Design review of the part built by this model. Coordinates are the model's own, in mm. Round coordinates to 2 decimals unless told otherwise and drop trailing zeros. Loops run counter-clockwise (first coordinate to the right, second up) from the corner with the lowest first, then second, coordinate; pieces in that order, holes last. Notation, with made-up numbers: M 37,-2.75 L 79,-2.75 A30 ccw 79,34.25 Z; hole C 58,45 d9. An arc over 180 degrees is marked long. Use a Markdown table: item, result.
from build123d import *

# Parameters (mm, degrees)
BOSS_EXTRUDE1_DEPTH = 3
FILLET1_R           = 5
CUT_EXTRUDE1_DEPTH  = 3
SKETCH3_W           = 3
SKETCH3_H           = 185.5
BOSS_EXTRUDE2_DEPTH = 5
BOSS_EXTRUDE3_DEPTH = 3
BOSS_EXTRUDE4_DEPTH = 3


with BuildPart() as part:
    # Sketch1 → Boss-Extrude1 (new body)
    with BuildSketch(Plane.XY):
        with BuildLine():
            Line((-23.5, 139.962429423), (-23.5, 114.5))
            Line((-23.5, 114.5), (3, 114.5))
            Line((3, 114.5), (3, 54.962429423))
            Line((3, 54.962429423), (-23.5, 54.962429423))
            Line((-23.5, 54.962429423), (-23.5, 29.5))
            Line((-23.5, 29.5), (3, 29.5))
            Line((3, 29.5), (3, -30.037570577))
            Line((3, -30.037570577), (-23.5, -30.037570577))
            Line((-23.5, -30.037570577), (-23.5, -55.5))
            Line((-23.5, -55.5), (3, -55.5))
            Line((3, -55.5), (3, -75.25))
            ThreePointArc((3, -75.25), (-20, -98.25), (-43, -75.25))
            Line((-43, -75.25), (-43, 160.25))
            ThreePointArc((-43, 160.25), (-20, 183.25), (3, 160.25))
            Line((3, 160.25), (3, 139.962429423))
            Line((3, 139.962429423), (-23.5, 139.962429423))
        make_face()
    extrude(amount=BOSS_EXTRUDE1_DEPTH)

    # Fillet1
    fillet1_edges = [part.edges().sort_by_distance(p)[0] for p in [
        (-23.5, 139.962429423, 1.5),
        (-23.5, 114.5, 1.5),
        (-23.5, 54.962429423, 1.5),
        (-23.5, 29.5, 1.5),
        (-23.5, -30.037570577, 1.5),
        (-23.5, -55.5, 1.5),
    ]]
    fillet(fillet1_edges, radius=FILLET1_R)

    # Sketch2 → Cut-Extrude1 (cut)
    with BuildSketch(Plane.XY.offset(3)):
        with BuildLine():
            Line((-31.934718262, 161.5), (-8.065281738, 161.5))
            ThreePointArc((-8.065281738, 161.5), (-8, 160.25), (-8.065281738, 159))
            Line((-8.065281738, 159), (-31.934718262, 159))
            ThreePointArc((-31.934718262, 159), (-32, 160.25), (-31.934718262, 161.5))
        make_face()
        with BuildLine():
            Line((-31.399013115, 164), (-8.600986885, 164))
            ThreePointArc((-8.600986885, 164), (-9.106587826, 165.283246588), (-9.756099376, 166.5))
            Line((-9.756099376, 166.5), (-30.243900624, 166.5))
            ThreePointArc((-30.243900624, 166.5), (-30.893412174, 165.283246588), (-31.399013115, 164))
        make_face()
        with BuildLine():
            Line((-28.212033853, 169), (-11.787966147, 169))
            ThreePointArc((-11.787966147, 169), (-20, 172.25), (-28.212033853, 169))
        make_face()
        with BuildLine():
            Line((-28.212033853, 151.5), (-11.787966147, 151.5))
            ThreePointArc((-11.787966147, 151.5), (-20, 148.25), (-28.212033853, 151.5))
        make_face()
        with BuildLine():
            Line((-30.243900624, 154), (-9.756099376, 154))
            ThreePointArc((-9.756099376, 154), (-9.106587826, 155.216753412), (-8.600986885, 156.5))
            Line((-8.600986885, 156.5), (-31.399013115, 156.5))
            ThreePointArc((-31.399013115, 156.5), (-30.893412174, 155.216753412), (-30.243900624, 154))
        make_face()
        with BuildLine():
            Line((-31.399013115, -71.5), (-8.600986885, -71.5))
            ThreePointArc((-8.600986885, -71.5), (-9.106587826, -70.216753412), (-9.756099376, -69))
            Line((-9.756099376, -69), (-30.243900624, -69))
            ThreePointArc((-30.243900624, -69), (-30.893412174, -70.216753412), (-31.399013115, -71.5))
        make_face()
        with BuildLine():
            Line((-28.212033853, -66.5), (-11.787966147, -66.5))
            ThreePointArc((-11.787966147, -66.5), (-20, -63.25), (-28.212033853, -66.5))
        make_face()
        with BuildLine():
            Line((-31.934718262, -74), (-8.065281738, -74))
            ThreePointArc((-8.065281738, -74), (-8, -75.25), (-8.065281738, -76.5))
            Line((-8.065281738, -76.5), (-31.934718262, -76.5))
            ThreePointArc((-31.934718262, -76.5), (-32, -75.25), (-31.934718262, -74))
        make_face()
        with BuildLine():
            Line((-28.212033853, -84), (-11.787966147, -84))
            ThreePointArc((-11.787966147, -84), (-20, -87.25), (-28.212033853, -84))
        make_face()
        with BuildLine():
            Line((-30.243900624, -81.5), (-9.756099376, -81.5))
            ThreePointArc((-9.756099376, -81.5), (-9.106587826, -80.283246588), (-8.600986885, -79))
            Line((-8.600986885, -79), (-31.399013115, -79))
            ThreePointArc((-31.399013115, -79), (-30.893412174, -80.283246588), (-30.243900624, -81.5))
        make_face()
    extrude(amount=-CUT_EXTRUDE1_DEPTH, mode=Mode.SUBTRACT)

    # Sketch3 → Boss-Extrude2 (add)
    with BuildSketch(Plane.XY.offset(3)):
        with Locations((-38.5, 42.5)):
            Rectangle(SKETCH3_W, SKETCH3_H)
    extrude(amount=BOSS_EXTRUDE2_DEPTH)

    # Sketch4 → Boss-Extrude3 (add)
    with BuildSketch(Plane.XZ.offset(30.037570577)):
        Polygon((-37, 8), (-37, 3), (-32, 3), align=None)
    extrude(amount=-BOSS_EXTRUDE3_DEPTH)

    # Sketch5 → Boss-Extrude4 (add)
    with BuildSketch(Plane(origin=(0, 114.5, 0), x_dir=(1, 0, 0), z_dir=(0, 1, 0))):
        Polygon((-37, -8), (-32, -3), (-37, -3), align=None)
    extrude(amount=-BOSS_EXTRUDE4_DEPTH)


solid = part.part
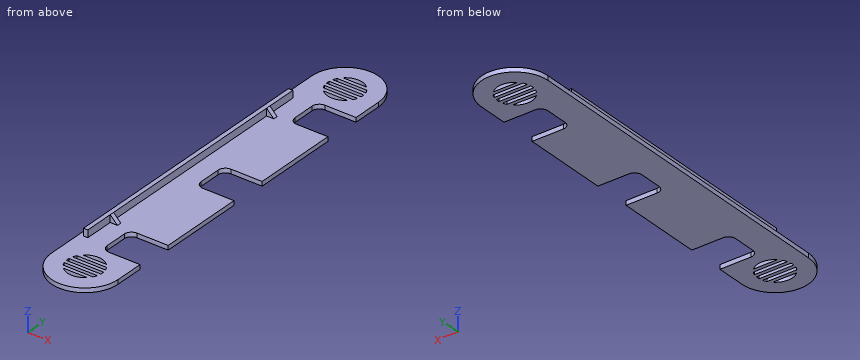
1. Take a section at B-B on z = 1.25. Count the separate pieces of the cut face and the enclosed holes in it, and give its area (3 significant figures).
Check values:
| item | result |
|---|---|
| separate pieces | 1 |
| enclosed holes | 10 |
| area | 10,000 mm² |
2. Take a section at C-C on y = 38. Give the boundary of the cut face in (x, z).
Check values:
| item | result |
|---|---|
| outline | M -43,0 L -23.5,0 L -23.5,3 L -37,3 L -37,8 L -40,8 L -40,3 L -43,3 Z |
3. Insertion check: pin 1 (1.5 mm diameter, centred on x = -38, z = 5, fed in from +Y); pin 2 (3 mm diameter, centred on x = -4.5, z = 1.5, fed in from -Y); pin 3 (5 mm diameter, centred on x = -22, y = 32, fed in from +Z). Each pin has a flat end and moves straight along its axis. Give the tip position at first contact, or say it passes through.
Check values:
| item | result |
|---|---|
| pin 1 | stops at y = 135.25 |
| pin 2 | stops at y = -93.5 |
| pin 3 | stops at z = 3 |
4. Wall thickness on line 1 along Y through (x, z) = (-1.5, 1.75); line 2 along X through (y, z) = (-11, 4.75); line 3 along Z through (x, y) = (-31.5, 3): over which ranges is each line inside the solid? List them lowest first. Write a range as from..to.
Check values:
| item | result |
|---|---|
| line 1 | y = -88.92..-55.5, -30.04..29.5, 54.96..114.5, 139.96..173.92 |
| line 2 | x = -40..-37 |
| line 3 | z = 0..3 |
5. Take a section at A-A on y = 105. Give the boundary of the cut face in (x, z).
Check values:
| item | result |
|---|---|
| outline | M -43,0 L 3,0 L 3,3 L -37,3 L -37,8 L -40,8 L -40,3 L -43,3 Z |
